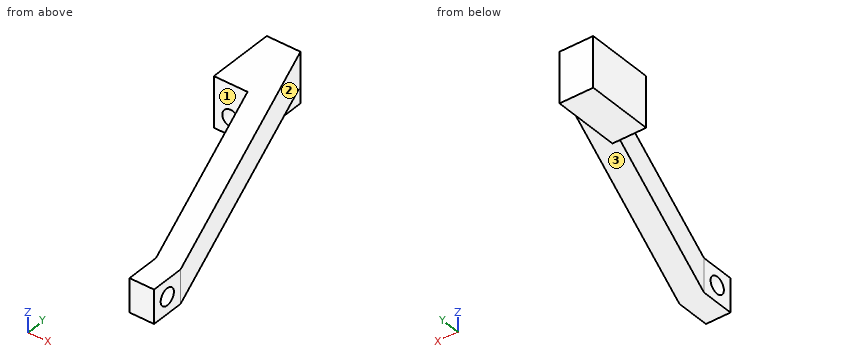
```python
from build123d import *

# Parameters (mm, degrees)
BOSS_EXTRUDE1_DEPTH = 12.7
SKETCH2_R           = 3.175
CUT_EXTRUDE1_DEPTH  = 10.24484395
SKETCH5_W           = 12.7
SKETCH5_H           = 25.4
BOSS_EXTRUDE2_DEPTH = 6.35
SKETCH4_R           = 3.175
CUT_EXTRUDE2_DEPTH  = 19.05


with BuildPart() as part:
    # Sketch1 → Boss-Extrude1 (new body)
    with BuildSketch(Plane.XY):
        Polygon((0, 0), (0, 25.4), (12.7, 25.4), (51.754006137, -81.9), (51.754006137, -94.6), (42.509162186, -94.6), (42.509162186, -81.9), (12.7, 0), align=None)
    extrude(amount=-BOSS_EXTRUDE1_DEPTH)

    # Sketch2 → Cut-Extrude1 (cut, through all)
    with BuildSketch(Plane.ZY.offset(-42.509162186)):
        with Locations((-6.35, -88.25)):
            Circle(SKETCH2_R)
    extrude(amount=-CUT_EXTRUDE1_DEPTH, mode=Mode.SUBTRACT)

    # Sketch5 → Boss-Extrude2 (add)
    with BuildSketch(Plane.XY.offset(-12.7)):
        with Locations((6.35, 12.7)):
            Rectangle(SKETCH5_W, SKETCH5_H)
    extrude(amount=-BOSS_EXTRUDE2_DEPTH)

    # Sketch4 → Cut-Extrude2 (cut)
    with BuildSketch(Plane.XZ):
        with Locations((6.35, -12.7)):
            Circle(SKETCH4_R)
    extrude(amount=-CUT_EXTRUDE2_DEPTH, mode=Mode.SUBTRACT)


solid = part.part
```
Input: part model. Units: mm. Frame: model coordinates. Face numbers are marked on the shaded views. A direction names the side the tool comes from. Coordinates: 2 decimals unless noted, no trailing zeros. Order: outer loops, then holes, each group sorted by start corner. A loop starts at its lowest first (then second) coordinate and runs counter-clockwise, first axis right, second up. Notation, with made-up numbers: (-33.75, 87.5) - (7.25, 87.5) arc R6 ccw to (7.25, 96.5) - close; hole circle Ø4 at (19, 42). An arc over 180 degrees is marked (long way). Return JSON: item names as keys, results as strings.
Q1. Cut plane C-C (x = 6.35). Return loops of the section in (y, z) (3 decimals).
The answers:
{"outline": "(0, -19.05) - (25.4, -19.05) - (25.4, 0) - (0, 0) - (0, -9.525) - (19.05, -9.525) - (19.05, -15.875) - (0, -15.875) - close"}
Q2. Cut plane D-D (z = -14). Return loops of the section in (x, y).
The answers:
{"outline": "(0, 0) - (3.45, 0) - (3.45, 19.05) - (9.25, 19.05) - (9.25, 0) - (12.7, 0) - (12.7, 25.4) - (0, 25.4) - close"}
Q3. First-contact query: pin 1 (1.9 mm diameter, centred on x = 7, z = -14, fed in from -Y); pin 2 (6.5 mm diameter, centred on x = 8, z = -12.5, fed in from -Y); pin 3 (4 mm diameter, centred on y = -88.5, z = -5, fed in from -X). Flat tips, straight axial feed; report the tip coordinate or a pass-through.
The answers:
{"pin 1": "stops at y = 19.05", "pin 2": "stops at y = 0", "pin 3": "stops at x = 42.51"}
Q4. Access query for the marked faces 1, 2 and 3. Directions: +Z, -Z, +X, -X, +Y, -Y. A direction counts if a zero-diameter tool reaches every point of the face in a straight line with its end or side. Return the directions, or none.
The answers:
{"face 1": "+Z, -Z, -X, -Y", "face 2": "+Z, -Z, +X, +Y", "face 3": "-Z, +X, +Y, -Y"}
Q5. Cut plane A-A (z = -6.35). Return loops of the section in (x, y) (3 decimals).
The answers:
{"outline": "(0, 0) - (12.7, 0) - (42.509, -81.9) - (42.509, -85.075) - (51.754, -85.075) - (51.754, -81.9) - (12.7, 25.4) - (0, 25.4) - close; (42.509, -94.6) - (51.754, -94.6) - (51.754, -91.425) - (42.509, -91.425) - close"}
Q6. Cut plane B-B (y = -88.25). Return loops of the section in (x, z) (3 decimals).
The answers:
{"outline": "(42.509, -12.7) - (51.754, -12.7) - (51.754, -9.525) - (42.509, -9.525) - close; (42.509, -3.175) - (51.754, -3.175) - (51.754, 0) - (42.509, 0) - close"}
Q7. Ray query, probe 1 along Z at (x, y) = (48, -88); probe 2 along Z at (x, y) = (6, 10); probe 3 along Y at (x, z) = (12.5, -16). Return the intervals inside material, ascending.
The answers:
{"probe 1": "z = -12.7 to -9.52, -3.18 to 0", "probe 2": "z = -19.05 to -15.86, -9.54 to 0", "probe 3": "y = 0 to 25.4"}
